Geometry: final body of the model. Coordinates: model frame, mm. A direction names the side the tool comes from. Give positions to 0.01 mm unless a question says otherwise; leave off trailing zeros. Order: outer loops, then holes, each group sorted by start corner. A loop starts at its lowest first (then second) coordinate and runs counter-clockwise, first axis right, second up. Notation, with made-up numbers: M 87,-23 L 96,-23 A9 ccw 96,-8 Z; hole C 67.25,54 d8. An arc over 180 degrees is marked long. Use CSV: the item, a comma, the result in double quotes.
```python
from build123d import *

# Parameters (mm, degrees)
SKETCH_R     = 1.5
PAD_DEPTH    = 4
CHAMFER_SIZE = 1.5


with BuildPart() as part:
    # Sketch → Pad (new body)
    with BuildSketch(Plane.XY):
        Polygon((-11.5, 35.58), (21.5, 35.58), (23.67, 33), (26.67, 33), (26.67, 27.5), (46.67, 23.6), (46.67, -23.6), (26.67, -27.5), (26.67, -33), (-26.67, -33), (-26.67, 33), (-13.67, 33), align=None)
        with Locations((43.17, 15.5)):
            Circle(SKETCH_R, mode=Mode.SUBTRACT)
        with Locations((43.17, -15.5)):
            Circle(SKETCH_R, mode=Mode.SUBTRACT)
        with Locations((19.05, 33)):
            Circle(SKETCH_R, mode=Mode.SUBTRACT)
        with Locations((-8.89, 33)):
            Circle(SKETCH_R, mode=Mode.SUBTRACT)
        with Locations((-24.13, -17.76)):
            Circle(SKETCH_R, mode=Mode.SUBTRACT)
        with Locations((24.17, -19)):
            Circle(SKETCH_R, mode=Mode.SUBTRACT)
        Polygon((8.660254, 13.222707), (8.660254, 23.222707), (0, 28.222707), (-8.660254, 23.222707), (-8.660254, 13.222707), (0, 8.222707), align=None, mode=Mode.SUBTRACT)
        Polygon((20.320508, -3.026554), (20.320508, 6.973446), (11.660254, 11.973446), (3, 6.973446), (3, -3.026554), (11.660254, -8.026554), align=None, mode=Mode.SUBTRACT)
        Polygon((0.418108, -5), (0.418108, 5), (-8.242146, 10), (-16.9024, 5), (-16.9024, -5), (-8.242146, -10), align=None, mode=Mode.SUBTRACT)
        Polygon((12.078362, -21.249261), (12.078362, -11.249261), (3.418108, -6.249261), (-5.242146, -11.249261), (-5.242146, -21.249261), (3.418108, -26.249261), align=None, mode=Mode.SUBTRACT)
        Polygon((26.67, 12.5), (26.67, -12.5), (37.17, -11), (37.17, 11), align=None, mode=Mode.SUBTRACT)
    extrude(amount=PAD_DEPTH)

    # Chamfer
    chamfer_edges = [part.edges().sort_by_distance(p)[0] for p in [
        (-26.67, 33, 2),
    ]]
    chamfer(chamfer_edges, length=CHAMFER_SIZE)


solid = part.part
```
1. Pin query (flat end, axial travel): pin 1 Ø5 at (x, y) = (-18, -2) entering from -Z; pin 2 Ø2 at (y, z) = (-30, 3) entering from +X; pin 3 Ø0.9 at (x, z) = (25, 1.5) entering from +Y. Return the tip coordinate at first contact, or that it passes through.
Answer:
pin 1,"z = 0"
pin 2,"x = 26.67"
pin 3,"y = 33"
2. Section A-A, the plane y = 15.5. Return the cut outline in (x, z), plus the area to 3 significant figures.
Answer:
outline,"M -26.67,0 L -8.66,0 L -8.66,4 L -26.67,4 Z; M 8.66,0 L 41.67,0 L 41.67,4 L 8.66,4 Z; M 44.67,0 L 46.67,0 L 46.67,4 L 44.67,4 Z"
area,"212 mm2"
3. Line query: line 1 (Y direction, x = 43.17, z = 1.7); line 2 (X direction, y = -3.5, z = 3.3); line 3 (Y direction, x = -24.13, z = 2.7). Output: solid intervals per line, ascending.
Answer:
line 1,"-24.28 to -17, -14 to 14, 17 to 24.28"
line 2,"-26.67 to -16.9, 0.42 to 3.82, 19.5 to 26.67, 37.17 to 46.67"
line 3,"-33 to -19.26, -16.26 to 33"
4. Section C-C, the plane x = 19. Return the cut outline in (y, z), plus the area to 3 significant figures.
Answer:
outline,"M -33,0 L -3.79,0 L -3.79,4 L -33,4 Z; M 7.74,0 L 31.5,0 L 31.5,4 L 7.74,4 Z; M 34.5,0 L 35.58,0 L 35.58,4 L 34.5,4 Z"
area,"216 mm2"
5. Section D-D, the plane z = 2.2. Give the number of separate pieces and of enclosed holes in the cut face, plus the area to 3 significant figures.
Answer:
separate pieces,"1"
enclosed holes,"11"
area,"3,300 mm2"
6. Reachability of faces 4 (the face through (2, 2, 4)), 5 (the face through (26.67, -30, 2)), 6 (the face through (-1, -23.7, 2)), 7 (the face through (25, 33, 2)) from +Z, -Z, +X, -X, +Y, -Y: full face, straight path, thin tool, end or side. Return the list, or none.
Answer:
face 4,"+Z, +X, -X, +Y, -Y"
face 5,"+Z, -Z, +X, -Y"
face 6,"+Z, -Z"
face 7,"+Z, -Z, +X, +Y"
7. Pull-direction query (Y, two-part tool) for faces 1 (the face through (-20, 33, 2)), 2 (the face through (-5.242, -16, 2)), 3 (the face through (2, 2, 0)); classes: +Y half, -Y half, draft (parallel to the pull), parting line (faces both ways), or undercut.
Answer:
face 1,"+Y half"
face 2,"undercut"
face 3,"draft"
8. Section B-B, the plane x = -24.13. Return the cut outline in (y, z).
Answer:
outline,"M -33,0 L -19.26,0 L -19.26,4 L -33,4 Z; M -16.26,0 L 33,0 L 33,4 L -16.26,4 Z"
